For this review, use the dimensioned drawing (mm, ordinates from the lowest corner) and the shaded views. Coordinates: 2 decimals unless noted, no trailing zeros. Write each loop counter-clockwise with the first axis right and the second up, starting at its lowest first coordinate (ties: lowest second). Pieces come first, ordered by that corner, then holes.
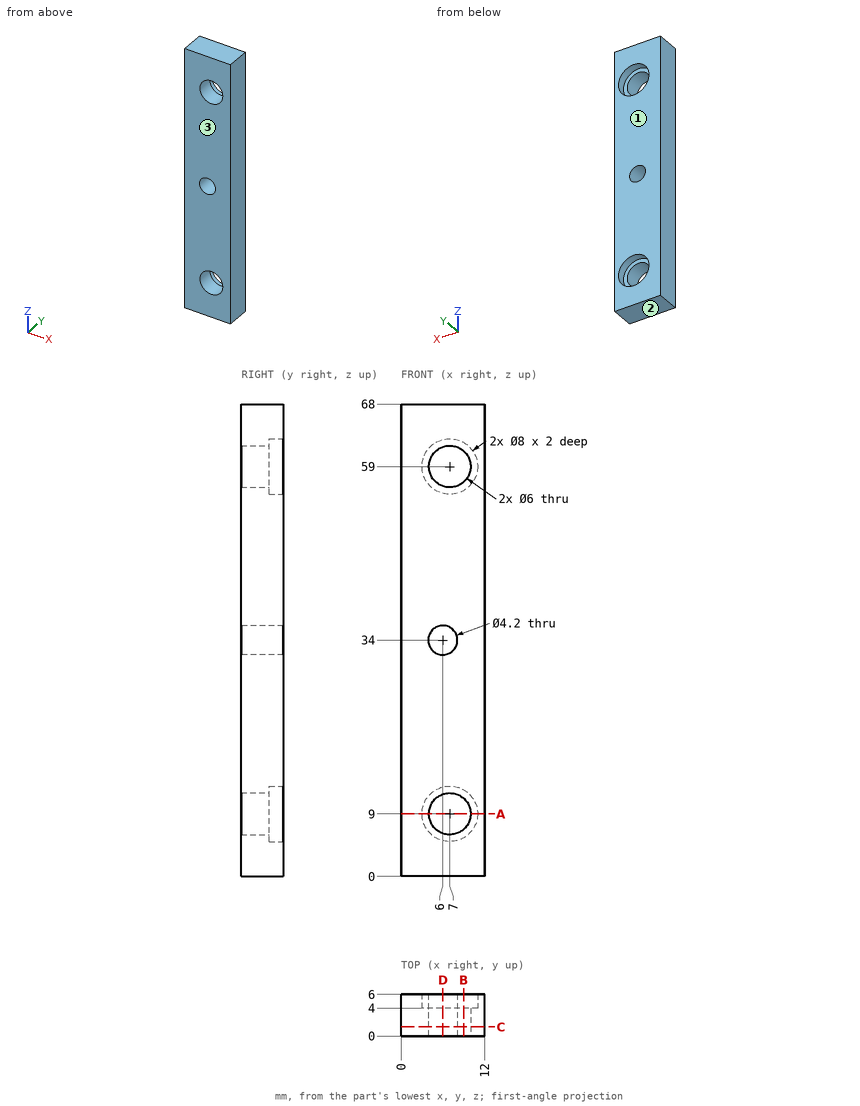
Item 1: Take a section at C-C, the plane y = 1.3. Write out the cut boundary in (x, z).
Solved:
outline: (0, 0) - (12, 0) - (12, 68) - (0, 68) - close; hole circle Ø4.2 at (6, 34); hole circle Ø6 at (7, 9); hole circle Ø6 at (7, 59)
Item 2: Take a section at B-B, the plane x = 9. Write out the cut boundary in (y, z).
Solved:
outline: (0, 0) - (6, 0) - (6, 5.54) - (4, 5.54) - (4, 6.76) - (0, 6.76) - close; (0, 11.24) - (4, 11.24) - (4, 12.46) - (6, 12.46) - (6, 55.54) - (4, 55.54) - (4, 56.76) - (0, 56.76) - close; (0, 61.24) - (4, 61.24) - (4, 62.46) - (6, 62.46) - (6, 68) - (0, 68) - close
Item 3: Take a section at D-D, the plane x = 6. Write out the cut boundary in (y, z), plus the area to 3 significant figures.
Solved:
outline: (0, 0) - (6, 0) - (6, 5.13) - (4, 5.13) - (4, 6.17) - (0, 6.17) - close; (0, 11.83) - (4, 11.83) - (4, 12.87) - (6, 12.87) - (6, 31.9) - (0, 31.9) - close; (0, 36.1) - (6, 36.1) - (6, 55.13) - (4, 55.13) - (4, 56.17) - (0, 56.17) - close; (0, 61.83) - (4, 61.83) - (4, 62.87) - (6, 62.87) - (6, 68) - (0, 68) - close
area: 307 mm2
Item 4: Take a section at A-A, the plane z = 9. Write out the cut boundary in (x, y).
Solved:
outline: (0, 0) - (4, 0) - (4, 4) - (3, 4) - (3, 6) - (0, 6) - close; (10, 0) - (12, 0) - (12, 6) - (11, 6) - (11, 4) - (10, 4) - close
Item 5: Mouldability with a two-part tool opening along Y and no side actions: class the marked faces 1, 2 and 3 as pulls with the +Y half, pulls with the -Y half, needs draft (parallel to the pull), parting line crosses it, or undercut.
Solved:
face 1: pulls with the +Y half
face 2: needs draft
face 3: pulls with the -Y half
Item 6: For pin 1 (5.5 mm diameter, centred on x = 6, z = 34, fed in from +Y), flat-tipped, find the tip position at first contact; note if it passes through.
Solved:
pin 1: stops at y = 6
Item 7: To check wall thickness, follow line 1 along X through (y, z) = (1.6, 9); line 2 along Z through (x, y) = (6, 3.5); line 3 along Z through (x, y) = (7, 3.15). State the ranges of each line that lie inside material, in increasing order.
Solved:
line 1: x = 0 to 4, 10 to 12
line 2: z = 0 to 6.17, 11.83 to 31.9, 36.1 to 56.17, 61.83 to 68
line 3: z = 0 to 6, 12 to 32.15, 35.85 to 56, 62 to 68
